The listing builds one solid part. Answer for the finished solid, in the listing's coordinates (mm). A direction names the side the tool comes from. Round coordinates to 2 decimals unless told otherwise and drop trailing zeros. Write each loop counter-clockwise with the first axis right and the second up, starting at its lowest first coordinate (ties: lowest second). Pieces come first, ordered by that corner, then holes.
from build123d import *

# Parameters (mm, degrees)
EXTRUDE_THIN1_DEPTH = 50.8
CUT_EXTRUDE1_DEPTH  = 55.250714281
LPATTERN1_COUNT     = 2
LPATTERN1_PITCH     = 25
FILLET1_R           = 0.25
FILLET2_R           = 1.25


with BuildPart() as part:
    # Sketch3 → Extrude-Thin1 (new body)
    with BuildSketch(Plane.XY):
        Polygon((-6.5, 17.5), (-6.5, 13.5), (0, 13.5), (0, -13.5), (-6.5, -13.5), (-6.5, -17.5), (-7.5, -17.5), (-7.5, -12.5), (-1, -12.5), (-1, 12.5), (-7.5, 12.5), (-7.5, 17.5), align=None)
    extrude(amount=EXTRUDE_THIN1_DEPTH)

    # Sketch4 → Cut-Extrude1 (cut, symmetric)
    with BuildSketch(Plane(origin=(0, 0, 0), x_dir=(0, 0, -1), z_dir=(1, 0, 0))):
        with BuildLine():
            Line((-6.65, -3.15), (-18.35, -3.15))
            ThreePointArc((-18.35, -3.15), (-21.5, 0), (-18.35, 3.15))
            Line((-18.35, 3.15), (-6.65, 3.15))
            ThreePointArc((-6.65, 3.15), (-3.5, 0), (-6.65, -3.15))
        make_face()
    cut_extrude1 = extrude(amount=CUT_EXTRUDE1_DEPTH, both=True, mode=Mode.SUBTRACT)

    # LPattern1: Cut-Extrude1 ×2
    with Locations(*[(0, 0, i * LPATTERN1_PITCH) for i in range(1, LPATTERN1_COUNT)]):
        add(cut_extrude1, mode=Mode.SUBTRACT)

    # Fillet1
    fillet1_edges = [part.edges().sort_by_distance(p)[0] for p in [
        (-6.5, 13.5, 25.4),
        (-6.5, -13.5, 25.4),
        (-1, -12.5, 25.4),
        (-1, 12.5, 25.4),
    ]]
    fillet(fillet1_edges, radius=FILLET1_R)

    # Fillet2
    fillet2_edges = [part.edges().sort_by_distance(p)[0] for p in [
        (0, 13.5, 25.4),
        (0, -13.5, 25.4),
        (-7.5, -12.5, 25.4),
        (-7.5, 12.5, 25.4),
    ]]
    fillet(fillet2_edges, radius=FILLET2_R)


solid = part.part
1. Section B-B on z = 11 is taken. Determine the outline of the cut face in (x, y), plus the area to 3 significant figures.
Geometry says:
outline: (-7.5, -17.5) - (-6.5, -17.5) - (-6.5, -13.75) arc R0.25 cw to (-6.25, -13.5) - (-1.25, -13.5) arc R1.25 ccw to (0, -12.25) - (0, -3.15) - (-1, -3.15) - (-1, -12.25) arc R0.25 cw to (-1.25, -12.5) - (-6.25, -12.5) arc R1.25 ccw to (-7.5, -13.75) - close; (-7.5, 13.75) arc R1.25 ccw to (-6.25, 12.5) - (-1.25, 12.5) arc R0.25 cw to (-1, 12.25) - (-1, 3.15) - (0, 3.15) - (0, 12.25) arc R1.25 ccw to (-1.25, 13.5) - (-6.25, 13.5) arc R0.25 cw to (-6.5, 13.75) - (-6.5, 17.5) - (-7.5, 17.5) - close
area: 40.4 mm2
2. Straight lines are drawn through the part: line 1 along Z through (x, y) = (-0.25, 0); line 2 along Y through (x, z) = (-3, 38); line 3 along X through (y, z) = (-3, 45). For each, find the intervals that lie inside material, in ascending order.
Geometry says:
line 1: z = 0 to 3.5, 21.5 to 28.5, 46.5 to 50.8
line 2: y = -13.5 to -12.5, 12.5 to 13.5
line 3: x = -1 to 0
3. Section A-A on x = -3 is taken. Determine the outline of the cut face in (y, z).
Geometry says:
outline: (-13.5, 0) - (-12.5, 0) - (-12.5, 50.8) - (-13.5, 50.8) - close; (12.5, 0) - (13.5, 0) - (13.5, 50.8) - (12.5, 50.8) - close
4. Section C-C on y = 0 is taken. Determine the outline of the cut face in (x, z).
Geometry says:
outline: (-1, 0) - (0, 0) - (0, 3.5) - (-1, 3.5) - close; (-1, 21.5) - (0, 21.5) - (0, 28.5) - (-1, 28.5) - close; (-1, 46.5) - (0, 46.5) - (0, 50.8) - (-1, 50.8) - close
5. For a pull along Z with two mould halves and no side action, classify faces 1 (the face through (-0.7, 0.1, 0)), 2 (the face through (-4, -12.5, 25)), 3 (the face through (-0.5, 0.1, 3.5)), 4 (the face through (-0.5, -3.15, 12.4)) as released by +Z, released by -Z, zero draft, split by the parting line, or undercut.
Geometry says:
face 1: released by -Z
face 2: zero draft
face 3: undercut
face 4: undercut
6. Given pin 1 (10 mm diameter, centred on y = -2, z = 16.5, fed in from -X); pin 2 (4 mm diameter, centred on y = -15, z = 36, fed in from +X); pin 3 (1.5 mm diameter, centred on x = -3.5, z = 33.5, fed in from +Y), each flat-ended and moving along its own axis, determine where each tip first touches the part or whether it passes through.
Geometry says:
pin 1: stops at x = -1
pin 2: stops at x = -0.25
pin 3: stops at y = 13.5
7. Section D-D on z = 23.5 is taken. Determine the outline of the cut face in (x, y), plus the area to 3 significant figures.
Geometry says:
outline: (-7.5, -17.5) - (-6.5, -17.5) - (-6.5, -13.75) arc R0.25 cw to (-6.25, -13.5) - (-1.25, -13.5) arc R1.25 ccw to (0, -12.25) - (0, 12.25) arc R1.25 ccw to (-1.25, 13.5) - (-6.25, 13.5) arc R0.25 cw to (-6.5, 13.75) - (-6.5, 17.5) - (-7.5, 17.5) - (-7.5, 13.75) arc R1.25 ccw to (-6.25, 12.5) - (-1.25, 12.5) arc R0.25 cw to (-1, 12.25) - (-1, -12.25) arc R0.25 cw to (-1.25, -12.5) - (-6.25, -12.5) arc R1.25 ccw to (-7.5, -13.75) - close
area: 46.7 mm2
8. A tool of negligible diameter and unlimited length cuts with its end or side. For faces 5 (the face through (-0.5, -0.1, 46.5)), 6 (the face through (-6.5, -16, 25)), 7 (the face through (-7.5, 16, 25)), 8 (the face through (-7.144, 12.876, 25.756)), from which of +Z, -Z, +X, -X, +Y, -Y can it reach the whole face along a straight path? Write none if from no direction.
Geometry says:
face 5: +X, -X
face 6: +Z, -Z, +X, -Y
face 7: +Z, -Z, -X, +Y, -Y
face 8: +Z, -Z, -X
